from build123d import *

# Parameters (mm, degrees)
F0_W = 3.2262087334
F0_H = 43.2004859692
F2_R = 5.08


with BuildPart() as f1:
    # F0 (on Front) → F1 (revolve)
    with BuildSketch(Plane.XZ):
        Polygon((0, -23.5666954911), (0, -38.8066954911), (20.32, -38.8066954911), (20.32, -23.5666954911), (3.2262087334, -23.5666954911), align=None)
        with Locations((1.6131043667, -1.9664525065)):
            Rectangle(F0_W, F0_H)
        Polygon((0, 34.8737904781), (0, 19.6337904781), (3.2262087334, 19.6337904781), (20.32, 19.6337904781), (20.32, 34.8737904781), align=None)
    revolve(axis=Axis((0, 0, -1.9664525065), (0, 0, 1)))

    # F2
    f2_edges = [f1.edges().sort_by_distance(p)[0] for p in [
        (-20.32, 0, 34.87379),
        (-20.32, 0, 19.63379),
        (-20.32, 0, -23.566695),
        (-20.32, 0, -38.806695),
    ]]
    fillet(f2_edges, radius=F2_R)


solid = f1.part
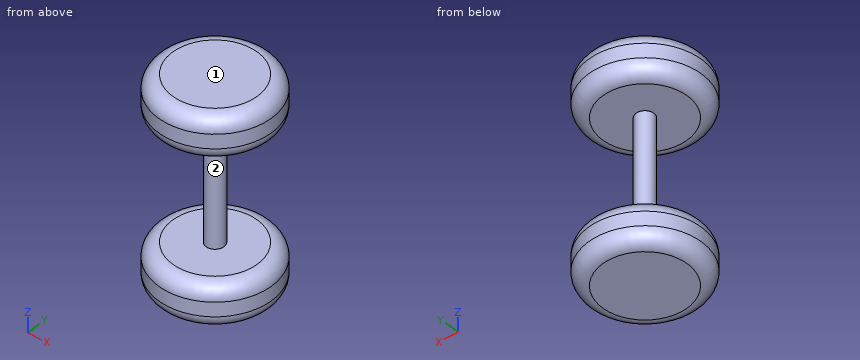
Geometry check sheet. Reference: the model listing, model coordinates, mm. Face numbers are marked on the shaded views. A direction names the side the tool comes from. Give positions to 0.01 mm unless a question says otherwise; leave off trailing zeros. Write each loop counter-clockwise with the first axis right and the second up, starting at its lowest first coordinate (ties: lowest second). Pieces come first, ordered by that corner, then holes. Notation, with made-up numbers: (77, 85) - (91, 85) arc R23 ccw to (91, 95) - close; hole circle Ø8 at (-29, 69). An arc over 180 degrees is marked (long way). Put each result on its own line as item: value.
1. Set-up check for the marked faces 1 and 2: record each of +Z, -Z, +X, -X, +Y, -Y from which the full face is reachable in a straight line by a thin tool's end or side.
Ans:
face 1: +Z, +X, -X, +Y, -Y
face 2: none
2. Sectioned sample at C-C, the plane z = 27.5. Enter the section's corners in (x, y), plus the area to 3 significant figures.
Ans:
outline: circle Ø40.64 at (0, 0)
area: 1,300 mm²
3. Sectioned sample at A-A, the plane y = 0. Enter the section's corners in (x, z), plus the area to 3 significant figures.
Ans:
outline: (-20.32, -33.73) arc R5.08 ccw to (-15.24, -38.81) - (15.24, -38.81) arc R5.08 ccw to (20.32, -33.73) - (20.32, -28.65) arc R5.08 ccw to (15.24, -23.57) - (3.23, -23.57) - (3.23, 19.63) - (15.24, 19.63) arc R5.08 ccw to (20.32, 24.71) - (20.32, 29.79) arc R5.08 ccw to (15.24, 34.87) - (-15.24, 34.87) arc R5.08 ccw to (-20.32, 29.79) - (-20.32, 24.71) arc R5.08 ccw to (-15.24, 19.63) - (-3.23, 19.63) - (-3.23, -23.57) - (-15.24, -23.57) arc R5.08 ccw to (-20.32, -28.65) - close
area: 1,470 mm²
4. Go/stop test with flat-tipped pins: pin 1 (5 mm diameter, centred on y = -15, z = -25, fed in from -X); pin 2 (12 mm diameter, centred on x = 4, z = 2, fed in from +Y); pin 3 (1 mm diameter, centred on x = 12.5, y = -15.5, fed in from +Z). Record where each tip stops, or that it passes through.
Ans:
pin 1: stops at x = -14.99
pin 2: stops at y = 3.23
pin 3: stops at z = 32.69
5. Sectioned sample at D-D, the plane z = 12. Enter the section's corners in (x, y).
Ans:
outline: circle Ø6.45 at (0, 0)
6. Thickness scan on line 1 (Z direction, x = 8, y = -9.5); line 2 (Z direction, x = 7, y = -14); line 3 (Y direction, x = 0, z = 16). Record the ranges inside material, lowest first.
Ans:
line 1: z = -38.81 to -23.57, 19.63 to 34.87
line 2: z = -38.79 to -23.58, 19.65 to 34.86
line 3: y = -3.23 to 3.23
